```python
from build123d import *

# Parameters (mm, degrees)
CROQUIS1_W              = 20
CROQUIS1_H              = 41
SALIENTE_EXTRUIR1_DEPTH = 1.5
SALIENTE_EXTRUIR3_DEPTH = 20
CROQUIS4_W              = 28
CROQUIS4_H              = 34
SALIENTE_EXTRUIR4_DEPTH = 1
SALIENTE_EXTRUIR5_DEPTH = 1
SALIENTE_EXTRUIR6_DEPTH = 1
SALIENTE_EXTRUIR7_DEPTH = 28


with BuildPart() as part:
    # Croquis1 → Saliente-Extruir1 (new body)
    with BuildSketch(Plane(origin=(0, 0, 0), x_dir=(1, 0, 0), z_dir=(0, 1, 0))):
        with Locations((42.14893617, 2.677304965)):
            Rectangle(CROQUIS1_W, CROQUIS1_H)
    extrude(amount=SALIENTE_EXTRUIR1_DEPTH)

    # Croquis3 → Saliente-Extruir3 (add)
    with BuildSketch(Plane(origin=(52.14893617, 0, 0), x_dir=(0, 0, -1), z_dir=(1, 0, 0))):
        Polygon((-17.822695035, 0), (-17.822695035, -3.5), (-14.822695035, -3.5), (-14.822695035, -2.5), (-16.822695035, -2.5), (-16.822695035, 0), align=None)
        Polygon((22.177304965, -2.5), (22.177304965, 0), (23.177304965, 0), (23.177304965, -3.5), (20.177304965, -3.5), (20.177304965, -2.5), align=None)
    extrude(amount=-SALIENTE_EXTRUIR3_DEPTH)

    # Croquis4 → Saliente-Extruir4 (add)
    with BuildSketch(Plane(origin=(52.14893617, 0, 0), x_dir=(0, 0, -1), z_dir=(1, 0, 0))):
        with Locations((2.677304965, 18.5)):
            Rectangle(CROQUIS4_W, CROQUIS4_H)
    extrude(amount=-SALIENTE_EXTRUIR4_DEPTH)

    # Croquis5 → Saliente-Extruir5 (add)
    with BuildSketch(Plane.XY.offset(11.322695035)):
        Polygon((51.14893617, 35.5), (32.14893617, 1.5), (51.14893617, 1.5), align=None)
    extrude(amount=-SALIENTE_EXTRUIR5_DEPTH)

    # Croquis6 → Saliente-Extruir6 (add)
    with BuildSketch(Plane(origin=(0, 0, -16.677304965), x_dir=(-1, 0, 0), z_dir=(0, 0, -1))):
        Polygon((-51.14893617, 35.5), (-32.14893617, 1.5), (-51.14893617, 1.5), align=None)
    extrude(amount=-SALIENTE_EXTRUIR6_DEPTH)

    # Croquis7 → Saliente-Extruir7 (add)
    with BuildSketch(Plane.XY.offset(11.322695035)):
        Polygon((52.14893617, 1.5), (52.14893617, 3.5), (33.266583229, 3.5), (32.14893617, 1.5), align=None)
    extrude(amount=-SALIENTE_EXTRUIR7_DEPTH)


solid = part.part
```
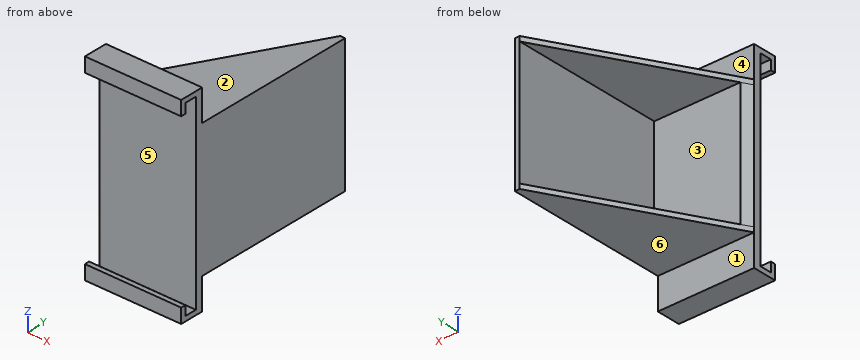
Geometry: final body of the model. Coordinates: model frame, mm. Face numbers are marked on the shaded views. A direction names the side the tool comes from. Round coordinates to 2 decimals unless told otherwise and drop trailing zeros. Loops run counter-clockwise (first coordinate to the right, second up) from the corner with the lowest first, then second, coordinate; pieces in that order, holes last.
Item 1: Section B-B, the plane y = 23.5. Output: boundary loops of the cut face in (x, z), plus the area to 3 significant figures.
Checked values:
outline: (44.44, -16.68) - (52.15, -16.68) - (52.15, 11.32) - (44.44, 11.32) - (44.44, 10.32) - (51.15, 10.32) - (51.15, -15.68) - (44.44, -15.68) - close
area: 41.4 mm2
Item 2: Mould query, pull axis Z, two halves, no side actions, for the marked faces 4, 5 and 6. Classes: released by +Z, released by -Z, zero draft, split by the parting line, or undercut.
Checked values:
face 4: zero draft
face 5: undercut
face 6: released by -Z
Item 3: Reachability of the marked faces 1, 2 and 3 from +Z, -Z, +X, -X, +Y, -Y: full face, straight path, thin tool, end or side. Return the list, or none.
Checked values:
face 1: -Z, +X, -X, +Y
face 2: +Z, +X, -X, +Y
face 3: -X, +Y
Item 4: Line query: L1, parallel to Z at x = 35.5, y = 6.5; L2, parallel to X at y = 11, z = 7; L3, parallel to Y at x = 41.5, z = -17. Output: solid intervals per line, ascending.
Checked values:
L1: z = -16.68 to -15.68, 10.32 to 11.32
L2: x = 51.15 to 52.15
L3: y = 0 to 1.5
Item 5: Contact query for flat-ended pins moving along their axis: P1, Ø1, axis at x = 37, y = 11, coming from the -Z side; P2, Ø1, axis at x = 35, z = 11, coming from the -Y side; P3, Ø12, axis at x = 43.5, y = 30, coming from the +Z side; P4, Ø2, axis at x = 35, y = 2, coming from the +Z side. Output: stop coordinate, or through.
Checked values:
P1: stops at z = -16.68
P2: stops at y = 0
P3: stops at z = 11.32
P4: stops at z = 17.82
Item 6: Section C-C, the plane x = 45.5. Output: boundary loops of the cut face in (y, z), plus the area to 3 significant figures.
Checked values:
outline: (-3.5, -23.18) - (1.5, -23.18) - (1.5, -16.68) - (25.39, -16.68) - (25.39, -15.68) - (3.5, -15.68) - (3.5, 10.32) - (25.39, 10.32) - (25.39, 11.32) - (1.5, 11.32) - (1.5, 17.82) - (-3.5, 17.82) - (-3.5, 14.82) - (-2.5, 14.82) - (-2.5, 16.82) - (0, 16.82) - (0, -22.18) - (-2.5, -22.18) - (-2.5, -20.18) - (-3.5, -20.18) - close
area: 172 mm2
Item 7: Section D-D, the plane y = 4. Output: boundary loops of the cut face in (x, z).
Checked values:
outline: (33.55, -16.68) - (52.15, -16.68) - (52.15, 11.32) - (33.55, 11.32) - (33.55, 10.32) - (51.15, 10.32) - (51.15, -15.68) - (33.55, -15.68) - close
Item 8: Section A-A, the plane z = -15. Output: boundary loops of the cut face in (x, y).
Checked values:
outline: (32.15, 0) - (52.15, 0) - (52.15, 35.5) - (51.15, 35.5) - (51.15, 3.5) - (33.27, 3.5) - (32.15, 1.5) - close
